Could you check a few things on this model? Use its own coordinates, in mm. Give positions to 0.01 mm unless a question says otherwise; leave off trailing zeros. Write each loop counter-clockwise with the first axis right and the second up, starting at its lowest first coordinate (ties: lowest second). Pieces come first, ordered by that corner, then holes. Notation, with made-up numbers: (28.5, 12.25) - (83.5, 12.25) arc R30 ccw to (83.5, 35.25) - close; hole circle Ø9 at (47.25, 71.5). An arc over 180 degrees is marked (long way). Write item = value, one per line.
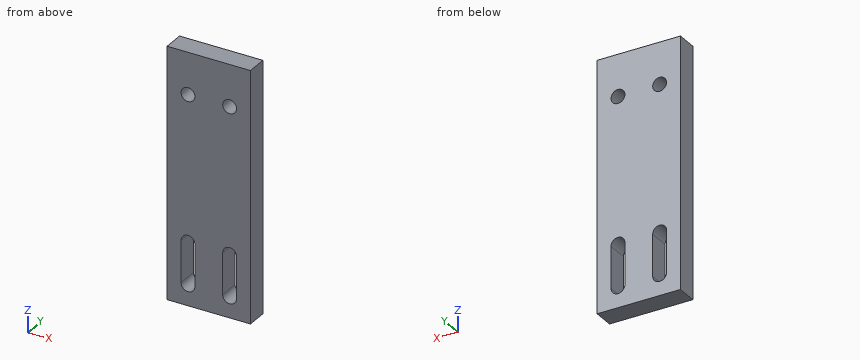
from build123d import *

# Parameters (mm, degrees)
F0_W     = 50.8
F0_H     = 152.4
F1_DEPTH = 12.7
F4_D     = 8.4328
F6_DEPTH = 12.701


with BuildPart() as f1:
    # F0 (on Front) → F1 (new body)
    with BuildSketch(Plane.XZ):
        with Locations((25.4, 76.2)):
            Rectangle(F0_W, F0_H)
    extrude(amount=F1_DEPTH)

    # F4 (through all)
    with Locations(Plane.XZ.offset(12.7)):
        with Locations((12.7, 127), (38.1, 127)):
            Hole(F4_D / 2)

    # F5 (on face) → F6 (cut, through all)
    with BuildSketch(Plane.XZ.offset(12.7)):
        with BuildLine():
            Line((16.9164, 12.7), (16.9164, 38.1))
            ThreePointArc((16.9164, 38.1), (12.7, 42.3164), (8.4836, 38.1))
            Line((8.4836, 38.1), (8.4836, 12.7))
            ThreePointArc((8.4836, 12.7), (12.7, 8.4836), (16.9164, 12.7))
        make_face()
        with BuildLine():
            Line((42.3164, 12.7), (42.3164, 38.1))
            ThreePointArc((42.3164, 38.1), (38.1, 42.3164), (33.8836, 38.1))
            Line((33.8836, 38.1), (33.8836, 12.7))
            ThreePointArc((33.8836, 12.7), (38.1, 8.4836), (42.3164, 12.7))
        make_face()
    extrude(amount=-F6_DEPTH, mode=Mode.SUBTRACT)


solid = f1.part
1. For pin 1 (3 mm diameter, centred on x = 15, z = 48, fed in from +Y), with a flat end and sliding along its axis, tell me the tip position at first contact or that it passes through.
Filled sheet:
pin_1 = 0
2. If we section it at A-A, the plane x = 38.1: Please give me the cut outline in (y, z), and give its area (3 significant figures).
Filled sheet:
outline = (-12.7, 0) - (0, 0) - (0, 8.48) - (-12.7, 8.48) - close; (-12.7, 42.32) - (0, 42.32) - (0, 122.78) - (-12.7, 122.78) - close; (-12.7, 131.22) - (0, 131.22) - (0, 152.4) - (-12.7, 152.4) - close
area = 1,400 mm2
3. If we section it at C-C, the plane y = -2: Please give me the cut outline in (x, z), and give its area (3 significant figures).
Filled sheet:
outline = (0, 0) - (50.8, 0) - (50.8, 152.4) - (0, 152.4) - close; hole (8.48, 12.7) arc R4.22 ccw to (16.92, 12.7) - (16.92, 38.1) arc R4.22 ccw to (8.48, 38.1) - close; hole circle Ø8.43 at (12.7, 127); hole (33.88, 12.7) arc R4.22 ccw to (42.32, 12.7) - (42.32, 38.1) arc R4.22 ccw to (33.88, 38.1) - close; hole circle Ø8.43 at (38.1, 127)
area = 7,090 mm2
4. If we section it at B-B, the plane z = 127: Please give me the cut outline in (x, y).
Filled sheet:
outline = (0, -12.7) - (8.48, -12.7) - (8.48, 0) - (0, 0) - close; (16.92, -12.7) - (33.88, -12.7) - (33.88, 0) - (16.92, 0) - close; (42.32, -12.7) - (50.8, -12.7) - (50.8, 0) - (42.32, 0) - close
5. I need wall thicknesses on line 1 (Z direction, x = 12.7, y = -6.5); line 2 (X direction, y = -4, z = 25); line 3 (X direction, y = -10.75, z = 128.5). Which ranges of each line are inside material? Lowest first, please.
Filled sheet:
line_1 = 0 to 8.48, 42.32 to 122.78, 131.22 to 152.4
line_2 = 0 to 8.48, 16.92 to 33.88, 42.32 to 50.8
line_3 = 0 to 8.76, 16.64 to 34.16, 42.04 to 50.8
